from build123d import *

# Parameters (mm, degrees)
SKETCH1_R           = 5.08
BOSS_EXTRUDE1_DEPTH = 7.62
SKETCH2_W           = 15.638324702
SKETCH2_H           = 10.16
CUT_EXTRUDE1_DEPTH  = 83.001098163
FILLET1_R           = 12.7
FILLET2_R           = 5.08


with BuildPart() as part:
    # Sketch1 → Boss-Extrude1 (new, symmetric)
    with BuildSketch(Plane(origin=(0, 0, 0), x_dir=(1, 0, 0), z_dir=(0, 1, 0))):
        with BuildLine():
            Line((2.735663722, 7.112), (8.018324702, 5.08))
            Line((8.018324702, 5.08), (8.018324702, 3.81))
            Line((8.018324702, 3.81), (63.101675298, 3.81))
            Line((63.101675298, 3.81), (63.101675298, 5.08))
            Line((63.101675298, 5.08), (68.384336278, 7.112))
            ThreePointArc((68.384336278, 7.112), (78.74, 0), (68.384336278, -7.112))
            Line((68.384336278, -7.112), (63.101675298, -5.08))
            Line((63.101675298, -5.08), (63.101675298, -3.81))
            Line((63.101675298, -3.81), (8.018324702, -3.81))
            Line((8.018324702, -3.81), (8.018324702, -5.08))
            Line((8.018324702, -5.08), (2.735663722, -7.112))
            ThreePointArc((2.735663722, -7.112), (-7.62, 0), (2.735663722, 7.112))
        make_face()
        with Locations(Location((0, 0, 0), (0, 0, 90))):
            Circle(SKETCH1_R, mode=Mode.SUBTRACT)
        with Locations(Location((71.12, 0, 0), (0, 0, 90))):
            Circle(SKETCH1_R, mode=Mode.SUBTRACT)
    extrude(amount=BOSS_EXTRUDE1_DEPTH, both=True)

    # Sketch2 → Cut-Extrude1 (cut, through all)
    with BuildSketch(Plane.XY.offset(13.97)):
        Polygon((8.018324702, 7.62), (63.101675298, 5.08), (78.74, 5.08), (78.74, 7.62), align=None)
        with Locations((0.199162351, 0)):
            Rectangle(SKETCH2_W, SKETCH2_H)
        Polygon((63.101675298, -5.08), (78.74, -5.08), (78.74, -7.62), (8.018324702, -7.62), align=None)
    extrude(amount=-CUT_EXTRUDE1_DEPTH, mode=Mode.SUBTRACT)

    # Fillet1
    # the kernel refuses this fillet: 12.7 mm, written as the material it adds along each edge
    with BuildSketch(Plane(origin=(63.101675298, 18.919504146, 3.81), x_dir=(-1, 0, 0), z_dir=(0, -1, 0))) as fillet1_piece_1_section:
        with BuildLine():
            CenterArc((5.535801658, -12.7), FILLET1_R, 90, 25.841932763)
            Line((0, -1.27), (0, 0))
            Line((0, 0), (5.535801658, 0))
        make_face()
    fillet1_piece_1 = extrude(amount=37.839008291, mode=Mode.PRIVATE)
    fillet1_piece_1 = split(fillet1_piece_1, bisect_by=Plane(origin=(59.36502655, 5.252304112, 3.912132652), z_dir=(-0.04606299102663346, -0.9989385370770718, 0)), keep=Keep.TOP, mode=Mode.PRIVATE)
    fillet1_piece_1 = split(fillet1_piece_1, bisect_by=Plane(origin=(59.844275634, -5.230205009, 3.912132652), z_dir=(-0.04606299102663346, 0.9989385370770718, 0)), keep=Keep.TOP, mode=Mode.PRIVATE)
    add(fillet1_piece_1)
    with BuildSketch(Plane(origin=(63.101675298, 18.919504146, -3.81), x_dir=(0, 0, -1), z_dir=(0, -1, 0))) as fillet1_piece_2_section:
        with BuildLine():
            CenterArc((12.7, -5.535801658), FILLET1_R, 154.158067237, 25.841932763)
            Line((0, -5.535801658), (0, 0))
            Line((0, 0), (1.27, 0))
        make_face()
    fillet1_piece_2 = extrude(amount=37.839008291, mode=Mode.PRIVATE)
    fillet1_piece_2 = split(fillet1_piece_2, bisect_by=Plane(origin=(62.135782482, 5.124539189, -4.63296), z_dir=(-0.04606299102663346, -0.9989385370770718, 0)), keep=Keep.TOP, mode=Mode.PRIVATE)
    fillet1_piece_2 = split(fillet1_piece_2, bisect_by=Plane(origin=(62.604689444, -5.10291698, -4.63296), z_dir=(-0.04606299102663346, 0.9989385370770718, 0)), keep=Keep.TOP, mode=Mode.PRIVATE)
    add(fillet1_piece_2)
    with BuildSketch(Plane(origin=(8.018324702, 8.759504146, -3.81), x_dir=(1, 0, 0), z_dir=(0, -1, 0))) as fillet1_piece_3_section:
        with BuildLine():
            CenterArc((5.535801658, -12.7), FILLET1_R, 90, 25.841932763)
            Line((0, -1.27), (0, 0))
            Line((0, 0), (5.535801658, 0))
        make_face()
    fillet1_piece_3 = extrude(amount=30.219008291, mode=Mode.PRIVATE)
    fillet1_piece_3 = split(fillet1_piece_3, bisect_by=Plane(origin=(11.809644031, 7.445174921, -3.912132652), z_dir=(-0.04606299102663346, -0.9989385370770718, 0)), keep=Keep.TOP, mode=Mode.PRIVATE)
    fillet1_piece_3 = split(fillet1_piece_3, bisect_by=Plane(origin=(11.757033309, 5.08, -3.912132652), z_dir=(0, 1, 0)), keep=Keep.TOP, mode=Mode.PRIVATE)
    add(fillet1_piece_3)
    with BuildSketch(Plane(origin=(8.018324702, -5.08, -3.81), x_dir=(1, 0, 0), z_dir=(0, -1, 0))) as fillet1_piece_4_section:
        with BuildLine():
            CenterArc((5.535801658, -12.7), FILLET1_R, 90, 25.841932763)
            Line((0, -1.27), (0, 0))
            Line((0, 0), (5.535801658, 0))
        make_face()
    fillet1_piece_4 = extrude(amount=16.379504146, mode=Mode.PRIVATE)
    fillet1_piece_4 = split(fillet1_piece_4, bisect_by=Plane(origin=(11.809644031, -7.445174921, -3.912132652), z_dir=(-0.04606299102663346, 0.9989385370770718, 0)), keep=Keep.TOP, mode=Mode.PRIVATE)
    add(fillet1_piece_4)
    with BuildSketch(Plane(origin=(8.018324702, 21.459504146, -3.81), x_dir=(1, 0, 0), z_dir=(0, -1, 0))) as fillet1_piece_5_section:
        with BuildLine():
            CenterArc((5.535801658, -12.7), FILLET1_R, 90, 25.841932763)
            Line((0, -1.27), (0, 0))
            Line((0, 0), (5.535801658, 0))
        make_face()
    fillet1_piece_5 = extrude(amount=16.379504146, mode=Mode.PRIVATE)
    fillet1_piece_5 = split(fillet1_piece_5, bisect_by=Plane(origin=(11.809644031, 7.445174921, -3.912132652), z_dir=(-0.04606299102663346, -0.9989385370770718, 0)), keep=Keep.TOP, mode=Mode.PRIVATE)
    add(fillet1_piece_5)
    with BuildSketch(Plane(origin=(8.018324702, 21.459504146, -3.81), x_dir=(1, 0, 0), z_dir=(0, -1, 0))) as fillet1_piece_6_section:
        with BuildLine():
            CenterArc((5.535801658, -12.7), FILLET1_R, 90, 25.841932763)
            Line((0, -1.27), (0, 0))
            Line((0, 0), (5.535801658, 0))
        make_face()
    fillet1_piece_6 = extrude(amount=30.219008291, mode=Mode.PRIVATE)
    fillet1_piece_6 = split(fillet1_piece_6, bisect_by=Plane(origin=(11.757033309, -5.08, -3.912132652), z_dir=(0, -1, 0)), keep=Keep.TOP, mode=Mode.PRIVATE)
    fillet1_piece_6 = split(fillet1_piece_6, bisect_by=Plane(origin=(11.809644031, -7.445174921, -3.912132652), z_dir=(-0.04606299102663346, 0.9989385370770718, 0)), keep=Keep.TOP, mode=Mode.PRIVATE)
    add(fillet1_piece_6)
    with BuildSketch(Plane(origin=(8.018324702, 8.759504146, 3.81), x_dir=(1, 0, 0), z_dir=(0, -1, 0))) as fillet1_piece_7_section:
        with BuildLine():
            CenterArc((5.535801658, 12.7), FILLET1_R, 244.158067237, 25.841932763)
            Line((0, 1.27), (0, 0))
            Line((0, 0), (5.535801658, 0))
        make_face()
    fillet1_piece_7 = extrude(amount=30.219008291, mode=Mode.PRIVATE)
    fillet1_piece_7 = split(fillet1_piece_7, bisect_by=Plane(origin=(11.809644031, 7.445174921, 3.912132652), z_dir=(-0.04606299102663346, -0.9989385370770718, 0)), keep=Keep.TOP, mode=Mode.PRIVATE)
    fillet1_piece_7 = split(fillet1_piece_7, bisect_by=Plane(origin=(11.757033309, 5.08, 3.912132652), z_dir=(0, 1, 0)), keep=Keep.TOP, mode=Mode.PRIVATE)
    add(fillet1_piece_7)
    with BuildSketch(Plane(origin=(8.018324702, -5.08, 3.81), x_dir=(1, 0, 0), z_dir=(0, -1, 0))) as fillet1_piece_8_section:
        with BuildLine():
            CenterArc((5.535801658, 12.7), FILLET1_R, 244.158067237, 25.841932763)
            Line((0, 1.27), (0, 0))
            Line((0, 0), (5.535801658, 0))
        make_face()
    fillet1_piece_8 = extrude(amount=16.379504146, mode=Mode.PRIVATE)
    fillet1_piece_8 = split(fillet1_piece_8, bisect_by=Plane(origin=(11.809644031, -7.445174921, 3.912132652), z_dir=(-0.04606299102663346, 0.9989385370770718, 0)), keep=Keep.TOP, mode=Mode.PRIVATE)
    add(fillet1_piece_8)
    with BuildSketch(Plane(origin=(8.018324702, 21.459504146, 3.81), x_dir=(0, 0, 1), z_dir=(0, -1, 0))) as fillet1_piece_9_section:
        with BuildLine():
            CenterArc((12.7, -5.535801658), FILLET1_R, 154.158067237, 25.841932763)
            Line((0, -5.535801658), (0, 0))
            Line((0, 0), (1.27, 0))
        make_face()
    fillet1_piece_9 = extrude(amount=16.379504146, mode=Mode.PRIVATE)
    fillet1_piece_9 = split(fillet1_piece_9, bisect_by=Plane(origin=(9.041953552, 7.572798491, 4.63296), z_dir=(-0.04606299102663346, -0.9989385370770718, 0)), keep=Keep.TOP, mode=Mode.PRIVATE)
    add(fillet1_piece_9)
    with BuildSketch(Plane(origin=(8.018324702, 21.459504146, 3.81), x_dir=(0, 0, 1), z_dir=(0, -1, 0))) as fillet1_piece_10_section:
        with BuildLine():
            CenterArc((12.7, -5.535801658), FILLET1_R, 154.158067237, 25.841932763)
            Line((0, -5.535801658), (0, 0))
            Line((0, 0), (1.27, 0))
        make_face()
    fillet1_piece_10 = extrude(amount=30.219008291, mode=Mode.PRIVATE)
    fillet1_piece_10 = split(fillet1_piece_10, bisect_by=Plane(origin=(8.985567945, -5.08, 4.63296), z_dir=(0, -1, 0)), keep=Keep.TOP, mode=Mode.PRIVATE)
    fillet1_piece_10 = split(fillet1_piece_10, bisect_by=Plane(origin=(9.041953552, -7.572798491, 4.63296), z_dir=(-0.04606299102663346, 0.9989385370770718, 0)), keep=Keep.TOP, mode=Mode.PRIVATE)
    add(fillet1_piece_10)

    # Fillet2
    # the kernel refuses this fillet: 5.08 mm, written as the material it takes off along each edge
    with BuildSketch(Plane(origin=(8.018324702, 5.08, -3.81), x_dir=(1, 0, 0), z_dir=(0, -1, 0)), Plane(origin=(8.018324702, 5.08, 3.81), x_dir=(0, 0, -1), z_dir=(0, -1, 0))) as fillet2_piece_1:
        with BuildLine():
            CenterArc((FILLET2_R, FILLET2_R), FILLET2_R, 180, 90)
            Line((0, FILLET2_R), (0, 0))
            Line((0, 0), (FILLET2_R, 0))
        make_face()
    extrude(amount=10.16, mode=Mode.SUBTRACT)


solid = part.part
Here's how the part is built. I have some questions about the finished solid (model axes, mm). A direction names the side the tool comes from. Coordinates: 2 decimals unless noted, no trailing zeros. Order: outer loops, then holes, each group sorted by start corner. A loop starts at its lowest first (then second) coordinate and runs counter-clockwise, first axis right, second up. Notation, with made-up numbers: M -21.75,72.25 L 23.25,72.25 A22 cw 23.25,104.25 Z; hole C 50,-21.5 d1. An arc over 180 degrees is marked long. Answer as CSV lines item,"result".
Item 1: For pin 1 (7.5 mm diameter, centred on x = 29, y = -1.5, fed in from -Z); pin 2 (1.5 mm diameter, centred on x = 20, z = 1.5, fed in from -Y); pin 3 (6 mm diameter, centred on x = 60, y = -1, fed in from +Z), each with a flat end and sliding along its axis, tell me the tip position at first contact or that it passes through.
Results found:
pin 1,"z = -3.81"
pin 2,"y = -7.1"
pin 3,"z = 5.03"
Item 2: Imagine slicing it at D-D on y = 1. Write out the boundary of the cut face in (x, z).
Results found:
outline,"M 8.18,0 A5.08 ccw 13.1,-3.81 L 57.57,-3.81 A12.7 cw 63.1,-5.08 L 68.38,-7.11 A7.62 ccw long 68.38,7.11 L 63.1,5.08 A12.7 cw 57.57,3.81 L 13.1,3.81 A5.08 ccw Z; hole C 71.12,0 d10.16"
Item 3: Imagine slicing it at C-C on z = -1.5. Write out the boundary of the cut face in (x, y), plus the area to 3 significant figures.
Results found:
outline,"M -7.47,-7.62 L -4.85,-7.62 L -4.85,-5.08 L -7.47,-5.08 Z; M -7.47,5.08 L -4.85,5.08 L -4.85,7.62 L -7.47,7.62 Z; M 4.85,-7.62 L 8.02,-7.62 L 63.1,-5.08 L 66.27,-5.08 L 66.27,5.08 L 63.1,5.08 L 8.02,7.62 L 4.85,7.62 L 4.85,5.08 L 8.84,5.08 L 8.84,-5.08 L 4.85,-5.08 Z; M 75.97,-5.08 L 78.59,-5.08 L 78.59,5.08 L 75.97,5.08 Z"
area,"779 mm2"
Item 4: If I drill on line 1 (X direction, y = 2.25, z = 0); line 2 (Z direction, x = 69, y = 0); line 3 (Y direction, x = 67, z = 3.5), over which ranges is the centre line in solid material (lowest first)?
Results found:
line 1,"8.18 to 66.04, 76.2 to 78.74"
line 2,"-7.32 to -4.62, 4.62 to 7.32"
line 3,"-5.08 to 5.08"
Item 5: On a 3-axis mill with a long thin cutter (end or side, diameter ignored), from which of +Z, -Z, +X, -X, +Y, -Y can I reach the whole of each face in a straight line? I mean faces 4 (the face through (5.34, 6.37, -6.11)), 5 (the face through (65.6, 5.08, 0.1)), 6 (the face through (9.951, 0.071, -2.717)). Say none if no direction works.
Results found:
face 4,"-Z, +X, +Y, -Y"
face 5,"+Z, -Z, +X, +Y"
face 6,"-Z, -X"
Item 6: Imagine slicing it at B-B on x = 0. Write out the boundary of the cut face in (y, z).
Results found:
outline,"M -7.62,-7.62 L -5.08,-7.62 L -5.08,-5.08 L -7.62,-5.08 Z; M -7.62,5.08 L -5.08,5.08 L -5.08,7.62 L -7.62,7.62 Z; M 5.08,-7.62 L 7.62,-7.62 L 7.62,-5.08 L 5.08,-5.08 Z; M 5.08,5.08 L 7.62,5.08 L 7.62,7.62 L 5.08,7.62 Z"
Item 7: We'd pull the mould along Z, two halves only. Please class faces 1 (the face through (78.737, 0.071, -0.207)), 2 (the face through (76.08, -0.07, 1.1)), 3 (the face through (65.78, 0.07, 6.11)): +Z half, -Z half, draft (parallel to the pull), parting line (faces both ways), or undercut.
Results found:
face 1,"parting line"
face 2,"undercut"
face 3,"+Z half"
Item 8: Imagine slicing it at A-A on x = 71.12. Write out the boundary of the cut face in (y, z).
Results found:
outline,"M -5.08,-7.62 L 5.08,-7.62 L 5.08,-5.08 L -5.08,-5.08 Z; M -5.08,5.08 L 5.08,5.08 L 5.08,7.62 L -5.08,7.62 Z"
